Verification items for the finished model (mm, model axes). Coordinates: 2 decimals unless noted, no trailing zeros. Write each loop counter-clockwise with the first axis right and the second up, starting at its lowest first coordinate (ties: lowest second). Pieces come first, ordered by that corner, then holes. Notation, with made-up numbers: (70, -33) - (95, -33) arc R14 cw to (95, -7) - close; hole circle Ø5 at (-16, 1.25). An arc over 180 degrees is marked (long way). Use CSV: the item, a comma, the result in double quotes. Start each with the question number.
```python
from build123d import *

# Parameters (mm, degrees)
BOSS_EXTRUDE1_DEPTH = 3.175
CUT_EXTRUDE1_REACH  = 5.175
SKETCH2_R           = 2.413
CUT_EXTRUDE2_REACH  = 5.175
SKETCH3_R           = 2.413
CUT_EXTRUDE3_REACH  = 5.175


with BuildPart() as part:
    # Sketch1 → Boss-Extrude1 (new body)
    with BuildSketch(Plane.XY):
        Polygon((315.214, 203.2), (518.414, 0), (127, 0), (0, 0), (0, 203.2), align=None)
    extrude(amount=BOSS_EXTRUDE1_DEPTH)

    # Sketch2 → Cut-Extrude1 (cut, up to next)
    with BuildSketch(Plane.XY.offset(3.175), mode=Mode.PRIVATE) as cut_extrude1_sk1:
        with Locations((12.7, 190.5)):
            Circle(SKETCH2_R)
    cut_extrude1_tool1 = extrude(cut_extrude1_sk1.sketch, amount=-CUT_EXTRUDE1_REACH, mode=Mode.PRIVATE) & part.part
    add(cut_extrude1_tool1.solids().sort_by_distance((12.7, 190.5, 3.175))[0], mode=Mode.SUBTRACT)
    # Sketch2 → Cut-Extrude1 (cut, up to next)
    with BuildSketch(Plane.XY.offset(3.175), mode=Mode.PRIVATE) as cut_extrude1_sk2:
        with Locations((83.82, 190.5)):
            Circle(SKETCH2_R)
    cut_extrude1_tool2 = extrude(cut_extrude1_sk2.sketch, amount=-CUT_EXTRUDE1_REACH, mode=Mode.PRIVATE) & part.part
    add(cut_extrude1_tool2.solids().sort_by_distance((83.82, 190.5, 3.175))[0], mode=Mode.SUBTRACT)
    # Sketch2 → Cut-Extrude1 (cut, up to next)
    with BuildSketch(Plane.XY.offset(3.175), mode=Mode.PRIVATE) as cut_extrude1_sk3:
        with Locations((154.94, 190.5)):
            Circle(SKETCH2_R)
    cut_extrude1_tool3 = extrude(cut_extrude1_sk3.sketch, amount=-CUT_EXTRUDE1_REACH, mode=Mode.PRIVATE) & part.part
    add(cut_extrude1_tool3.solids().sort_by_distance((154.94, 190.5, 3.175))[0], mode=Mode.SUBTRACT)
    # Sketch2 → Cut-Extrude1 (cut, up to next)
    with BuildSketch(Plane.XY.offset(3.175), mode=Mode.PRIVATE) as cut_extrude1_sk4:
        with Locations((226.06, 190.5)):
            Circle(SKETCH2_R)
    cut_extrude1_tool4 = extrude(cut_extrude1_sk4.sketch, amount=-CUT_EXTRUDE1_REACH, mode=Mode.PRIVATE) & part.part
    add(cut_extrude1_tool4.solids().sort_by_distance((226.06, 190.5, 3.175))[0], mode=Mode.SUBTRACT)
    # Sketch2 → Cut-Extrude1 (cut, up to next)
    with BuildSketch(Plane.XY.offset(3.175), mode=Mode.PRIVATE) as cut_extrude1_sk5:
        with Locations((12.7, 114.3)):
            Circle(SKETCH2_R)
    cut_extrude1_tool5 = extrude(cut_extrude1_sk5.sketch, amount=-CUT_EXTRUDE1_REACH, mode=Mode.PRIVATE) & part.part
    add(cut_extrude1_tool5.solids().sort_by_distance((12.7, 114.3, 3.175))[0], mode=Mode.SUBTRACT)
    # Sketch2 → Cut-Extrude1 (cut, up to next)
    with BuildSketch(Plane.XY.offset(3.175), mode=Mode.PRIVATE) as cut_extrude1_sk6:
        with Locations((12.7, 38.1)):
            Circle(SKETCH2_R)
    cut_extrude1_tool6 = extrude(cut_extrude1_sk6.sketch, amount=-CUT_EXTRUDE1_REACH, mode=Mode.PRIVATE) & part.part
    add(cut_extrude1_tool6.solids().sort_by_distance((12.7, 38.1, 3.175))[0], mode=Mode.SUBTRACT)

    # Sketch3 → Cut-Extrude2 (cut, up to next)
    with BuildSketch(Plane.XY.offset(3.175), mode=Mode.PRIVATE) as cut_extrude2_sk1:
        with Locations((481.403487758, 19.05)):
            Circle(SKETCH3_R)
    cut_extrude2_tool1 = extrude(cut_extrude2_sk1.sketch, amount=-CUT_EXTRUDE2_REACH, mode=Mode.PRIVATE) & part.part
    add(cut_extrude2_tool1.solids().sort_by_distance((481.403488, 19.05, 3.175))[0], mode=Mode.SUBTRACT)
    # Sketch3 → Cut-Extrude2 (cut, up to next)
    with BuildSketch(Plane.XY.offset(3.175), mode=Mode.PRIVATE) as cut_extrude2_sk2:
        with Locations((427.521951031, 72.931536726)):
            Circle(SKETCH3_R)
    cut_extrude2_tool2 = extrude(cut_extrude2_sk2.sketch, amount=-CUT_EXTRUDE2_REACH, mode=Mode.PRIVATE) & part.part
    add(cut_extrude2_tool2.solids().sort_by_distance((427.521951, 72.931537, 3.175))[0], mode=Mode.SUBTRACT)
    # Sketch3 → Cut-Extrude2 (cut, up to next)
    with BuildSketch(Plane.XY.offset(3.175), mode=Mode.PRIVATE) as cut_extrude2_sk3:
        with Locations((373.640414305, 126.813073453)):
            Circle(SKETCH3_R)
    cut_extrude2_tool3 = extrude(cut_extrude2_sk3.sketch, amount=-CUT_EXTRUDE2_REACH, mode=Mode.PRIVATE) & part.part
    add(cut_extrude2_tool3.solids().sort_by_distance((373.640414, 126.813073, 3.175))[0], mode=Mode.SUBTRACT)
    # Sketch3 → Cut-Extrude2 (cut, up to next)
    with BuildSketch(Plane.XY.offset(3.175), mode=Mode.PRIVATE) as cut_extrude2_sk4:
        with Locations((319.758877579, 180.694610179)):
            Circle(SKETCH3_R)
    cut_extrude2_tool4 = extrude(cut_extrude2_sk4.sketch, amount=-CUT_EXTRUDE2_REACH, mode=Mode.PRIVATE) & part.part
    add(cut_extrude2_tool4.solids().sort_by_distance((319.758878, 180.69461, 3.175))[0], mode=Mode.SUBTRACT)

    # Sketch4 → Cut-Extrude3 (cut, up to next)
    with BuildSketch(Plane.XY.offset(3.175), mode=Mode.PRIVATE) as cut_extrude3_sk1:
        Polygon((315.214, 203.2), (248.539, 203.2), (248.539, 174.625), (303.377847455, 174.625), (342.154768363, 135.848079092), (362.360344636, 156.053655364), align=None)
    cut_extrude3_tool1 = extrude(cut_extrude3_sk1.sketch, amount=-CUT_EXTRUDE3_REACH, mode=Mode.PRIVATE) & part.part
    add(cut_extrude3_tool1.solids().sort_by_distance((305.025183, 178.602019, 3.175))[0], mode=Mode.SUBTRACT)


solid = part.part
```
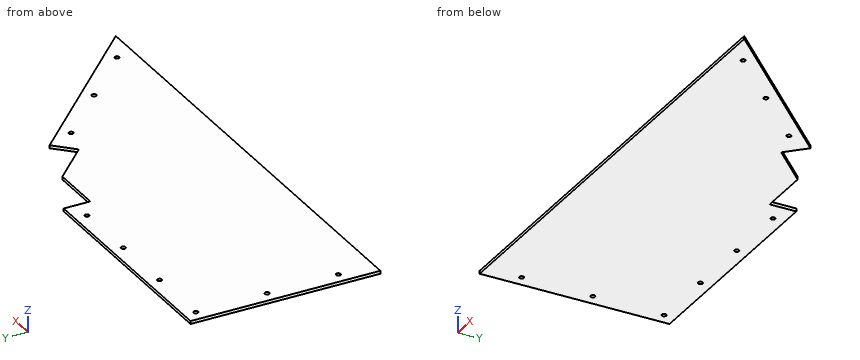
Q1. Cross-section at A-A (z = 2.4). State how many separate pieces and enclosed holes the cut face has, plus the area to 3 significant figures.
Q2. Cross-section at C-C (x = 418.5). Record the cut outline in (y, z) (3 decimals).
Q3. Cross-section at B-B (y = 180). Record the cut outline in (x, z) (3 decimals), plus the area to 3 significant figures.
Q4. Scan lines: line 1 along Y through (x, z) = (12.7, 2.3); line 2 along X through (y, z) = (190.5, 1.8); line 3 along X through (y, z) = (144, 1.45). Record each from-to range of solid material in increasing order. Write a range as from..to.
Q5. Gauge pin test, flat ends, axial feed: pin 1 (3 mm diameter, centred on x = 12.7, y = 190.5, fed in from -Z); pin 2 (6.5 mm diameter, centred on x = 427.52, y = 72.93, fed in from +Z) (3 decimals); pin 3 (1.6 mm diameter, centred on x = 267, z = 1, fed in from +Y) (3 decimals). Record the tip position at first contact, or that the pin passes through.
Reply:
1,separate pieces,"1"
1,enclosed holes,"9"
1,area,"81,100 mm^2"
2,outline,"(0, 0) - (99.914, 0) - (99.914, 3.175) - (0, 3.175) - close"
3,outline,"(0, 0) - (248.539, 0) - (248.539, 3.175) - (0, 3.175) - close"
3,area,"789 mm^2"
4,line 1,"0..35.69, 40.51..111.89, 116.71..188.09, 192.91..203.2"
4,line 2,"0..10.29, 15.11..81.41, 86.23..152.53, 157.35..223.65, 228.47..248.54"
4,line 3,"0..334, 350.31..374.41"
5,pin 1,"through"
5,pin 2,"z = 3.175"
5,pin 3,"y = 174.625"
